```python
from build123d import *

# Parameters (mm, degrees)
BOSS_EXTRUDE1_DEPTH     = 19
SKETCH3_W               = 256.5
SKETCH3_H               = 16.8
BOSS_EXTRUDE2_DEPTH     = 19
CUT_EXTRUDE1_DEPTH      = 19
CUT_EXTRUDE1_DEPTH_BACK = 19
SKETCH7_W               = 16
SKETCH7_H               = 5
HOLE1_D                 = 8.566
HOLE1_DEPTH             = 8.5
HOLE1_CSINK_D           = 9.728
HOLE1_CSINK_ANGLE       = 90
HOLE2_D                 = 8.566
HOLE2_DEPTH             = 8.5
HOLE2_CSINK_D           = 9.728
HOLE2_CSINK_ANGLE       = 90


with BuildPart() as part:
    # Sketch1 → Revolve1 (revolve)
    with BuildSketch(Plane.XY, mode=Mode.PRIVATE) as revolve1_sk:
        with BuildLine():
            Line((0, 0), (0, 13.3))
            Line((0, 13.3), (0.6, 13.9))
            Line((0.6, 13.9), (3, 13.9))
            Line((3, 13.9), (4.1, 15))
            Line((4.1, 15), (20.95, 15))
            Line((20.95, 15), (21.865685425, 14.084314575))
            ThreePointArc((21.865685425, 14.084314575), (22.125224104, 13.910896374), (22.43137085, 13.85))
            Line((22.43137085, 13.85), (23.2, 13.85))
            ThreePointArc((23.2, 13.85), (23.765685425, 14.084314575), (24, 14.65))
            Line((24, 14.65), (24, 15))
            Line((24, 15), (26, 15))
            Line((26, 15), (26, 0))
            Line((26, 0), (0, 0))
        make_face()
    revolve(revolve1_sk.sketch.rotate(Axis((26, 0, 0), (-1, 0, 0)), 270), axis=Axis((26, 0, 0), (-1, 0, 0)))

    # Sketch2 → Boss-Extrude1 (add)
    with BuildSketch(Plane(origin=(26, 0, 0), x_dir=(0, 0, -1), z_dir=(1, 0, 0))):
        with BuildLine():
            Line((8.6, 17.125419703), (8.6, 18.8))
            ThreePointArc((8.6, 18.8), (8.541421356, 18.941421356), (8.4, 19))
            Line((8.4, 19), (-8.4, 19))
            ThreePointArc((-8.4, 19), (-8.541421356, 18.941421356), (-8.6, 18.8))
            Line((-8.6, 18.8), (-8.6, 17.125419703))
            ThreePointArc((-8.6, 17.125419703), (-8.643579846, 16.969699747), (-8.761658031, 16.859221469))
            ThreePointArc((-8.761658031, 16.859221469), (0, -19), (8.761658031, 16.859221469))
            ThreePointArc((8.761658031, 16.859221469), (8.643579846, 16.969699747), (8.6, 17.125419703))
        make_face()
    extrude(amount=BOSS_EXTRUDE1_DEPTH)

    # Sketch3 → Revolve2 (revolve)
    with BuildSketch(Plane.XY, mode=Mode.PRIVATE) as revolve2_sk:
        with Locations((173.25, 8.4)):
            Rectangle(SKETCH3_W, SKETCH3_H)
    revolve(revolve2_sk.sketch.rotate(Axis((301.5, 0, 0), (-1, 0, 0)), 270), axis=Axis((301.5, 0, 0), (-1, 0, 0)))

    # Sketch4 → Boss-Extrude2 (add)
    with BuildSketch(Plane(origin=(301.5, 0, 0), x_dir=(0, 0, -1), z_dir=(1, 0, 0))):
        with BuildLine():
            Line((8.6, 17.125419703), (8.6, 18.8))
            ThreePointArc((8.6, 18.8), (8.541421356, 18.941421356), (8.4, 19))
            Line((8.4, 19), (-8.4, 19))
            ThreePointArc((-8.4, 19), (-8.541421356, 18.941421356), (-8.6, 18.8))
            Line((-8.6, 18.8), (-8.6, 17.125419703))
            ThreePointArc((-8.6, 17.125419703), (-8.643579846, 16.969699747), (-8.761658031, 16.859221469))
            ThreePointArc((-8.761658031, 16.859221469), (0, -19), (8.761658031, 16.859221469))
            ThreePointArc((8.761658031, 16.859221469), (8.643579846, 16.969699747), (8.6, 17.125419703))
        make_face()
    extrude(amount=BOSS_EXTRUDE2_DEPTH)

    # Sketch5 → Revolve3 (revolve)
    with BuildSketch(Plane.XY, mode=Mode.PRIVATE) as revolve3_sk:
        with BuildLine():
            Line((320.5, 0), (320.5, 15))
            Line((320.5, 15), (322.5, 15))
            Line((322.5, 15), (322.5, 14.65))
            ThreePointArc((322.5, 14.65), (322.734314575, 14.084314575), (323.3, 13.85))
            Line((323.3, 13.85), (324.06862915, 13.85))
            ThreePointArc((324.06862915, 13.85), (324.374775896, 13.910896374), (324.634314575, 14.084314575))
            Line((324.634314575, 14.084314575), (325.55, 15))
            Line((325.55, 15), (342.4, 15))
            Line((342.4, 15), (343.5, 13.9))
            Line((343.5, 13.9), (345.9, 13.9))
            Line((345.9, 13.9), (346.5, 13.3))
            Line((346.5, 13.3), (346.5, 0))
            Line((346.5, 0), (320.5, 0))
        make_face()
    revolve(revolve3_sk.sketch.rotate(Axis((346.5, 0, 0), (-1, 0, 0)), 270), axis=Axis((346.5, 0, 0), (-1, 0, 0)))

    # Sketch6 → Cut-Extrude1 (cut, two sides: drawn at the far end of the back side and taken through both)
    with BuildSketch(Plane(origin=(0, 0, 0), x_dir=(1, 0, 0), z_dir=(0, 1, 0)).offset(-CUT_EXTRUDE1_DEPTH_BACK)):
        Polygon((321.5, 24), (321.5, 8), (346.5, 8), (346.5, -8), (321.5, -8), (321.5, -24), (362.5, -24), (362.5, 24), align=None)
    extrude(amount=CUT_EXTRUDE1_DEPTH + CUT_EXTRUDE1_DEPTH_BACK, mode=Mode.SUBTRACT)

    # Sketch7 → Cut-Revolve1 (revolve, cut)
    with BuildSketch(Plane(origin=(334.5, 0, 0), x_dir=(0, 0, -1), z_dir=(1, 0, 0)), mode=Mode.PRIVATE) as cut_revolve1_sk:
        with Locations((0, 2.5)):
            Rectangle(SKETCH7_W, SKETCH7_H)
    revolve(cut_revolve1_sk.sketch.rotate(Axis((334.5, 0, -8), (0, 0, 1)), 270), axis=Axis((334.5, 0, -8), (0, 0, 1)), mode=Mode.SUBTRACT)

    # Hole1
    with Locations(Plane(origin=(0, 19, 0), x_dir=(1, 0, 0), z_dir=(0, 1, 0))):
        with Locations((35, 0)):
            CounterSinkHole(HOLE1_D / 2, HOLE1_CSINK_D / 2, depth=HOLE1_DEPTH, counter_sink_angle=HOLE1_CSINK_ANGLE)

    # Hole2
    with Locations(Plane(origin=(0, 19, 0), x_dir=(1, 0, 0), z_dir=(0, 1, 0))):
        with Locations((311.5, 0)):
            CounterSinkHole(HOLE2_D / 2, HOLE2_CSINK_D / 2, depth=HOLE2_DEPTH, counter_sink_angle=HOLE2_CSINK_ANGLE)

    # Sketch12 → Cut-Revolve2 (revolve, cut)
    with BuildSketch(Plane.XY, mode=Mode.PRIVATE) as cut_revolve2_sk:
        Polygon((-8, 0), (-8, 6), (57, 6), (57, 16), (290, 16), (290, 0), align=None)
    revolve(cut_revolve2_sk.sketch.rotate(Axis((290, 0, 0), (-1, 0, 0)), 270), axis=Axis((290, 0, 0), (-1, 0, 0)), mode=Mode.SUBTRACT)


solid = part.part
```
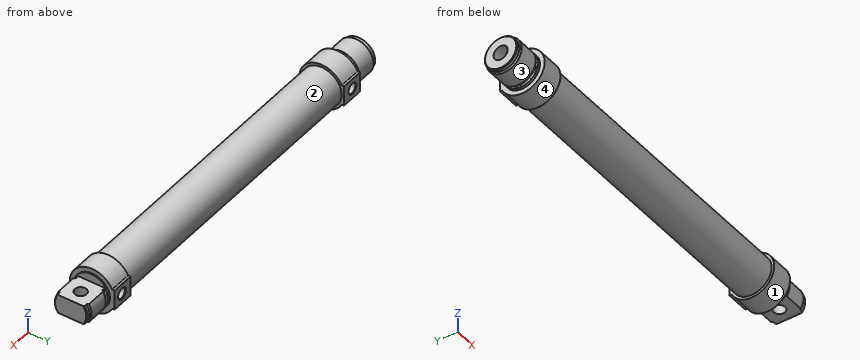
Work out the finished part from the listing and answer in its coordinate system (mm). Face numbers are marked on the shaded views. A direction names the side the tool comes from. Give positions to 0.01 mm unless a question says otherwise; leave off trailing zeros. Loops run counter-clockwise (first coordinate to the right, second up) from the corner with the lowest first, then second, coordinate; pieces in that order, holes last. Notation, with made-up numbers: M 73,21.5 L 81,21.5 A25 ccw 81,33.5 Z; hole C 36.25,-32 d6. An arc over 180 degrees is marked long. One line per item, written item: value. Start each with the question number.
1. Find section A-A (x = 334.5). Give the vertices of the cut face in (y, z).
2. Find section B-B (x = 35). Give the vertices of the cut face in (y, z).
3. Find section C-C (x = 155). Give the vertices of the cut face in (y, z), and give its area (3 significant figures).
4. Which of the six approach directions +Z, -Z, +X, -X, +Y, -Y give full straight-line access (tool end or side, diameter ignored) to the marked faces 3 and 4?
5. Determine the mould class of the marked faces 1 and 2 for opening direction X: released by +X, released by -X, zero draft, split by the parting line, or undercut.
6. Each of these flat-tipped pins is pushed along its axis until it touches: P1, Ø12, axis at x = 123, y = 10, coming from the +Z side; P2, Ø1.8, axis at x = 35, y = 18, coming from the +Z side; P3, Ø5, axis at x = 250.5, y = -2, coming from the -Z side; P4, Ø8, axis at x = 334.5, y = 0, coming from the -Z side. Where does it stop, or does it pass through?
7. Find the intervals of material crossed by probe 1 along Z at (x, y) = (311.5, 15.75); probe 2 along Y at (x, z) = (334, -3); probe 3 along X at (y, z) = (6, -3), in increasing order.
Reported:
1. outline: M -12.69,-8 L -5,-8 L -5,8 L -12.69,8 A15 ccw Z; M 5,-8 L 12.69,-8 A15 ccw 12.69,8 L 5,8 Z
2. outline: M 10.5,-4.28 L 10.5,4.28 L 18.42,4.28 L 19,4.86 L 19,8.4 A0.2 ccw 18.8,8.6 L 17.13,8.6 A0.3 cw 16.86,8.76 A19 ccw long 16.86,-8.76 A0.3 cw 17.13,-8.6 L 18.8,-8.6 A0.2 ccw 19,-8.4 L 19,-4.86 L 18.42,-4.28 Z; hole C 0,0 d12
3. outline: C 0,0 d33.6; hole C 0,0 d32
3. area: 82.4 mm²
4. face 3: -X
4. face 4: +X, -X
5. face 1: zero draft
5. face 2: undercut
6. P1: stops at z = 16.32
6. P2: stops at z = 8.6
6. P3: stops at z = -16.8
6. P4: passes through
7. probe 1: z = -10.63 to -4.28, 4.28 to 10.63
7. probe 2: y = -14.7 to -4.97, 4.97 to 14.7
7. probe 3: x = 0 to 57, 290 to 346.5
